```python
from build123d import *

# Parameters (mm, degrees)
SKETCH_1_R          = 32.5
SKETCH_1_R_2        = 13.625
SKETCH_1_R_3        = 2
SKETCH_1_R_4        = 1.65
SKETCH_1_R_5        = 1.4
EXTRUDE_1_DEPTH     = 4
SKETCH_2_R          = 1
CUT_EXTRUDE_1_DEPTH = 10


with BuildPart() as part:
    # 草图1 → 凸台-拉伸1 (new body)
    with BuildSketch(Plane.XY):
        with Locations((-0.261189045, 0.652972612)):
            Circle(SKETCH_1_R)
        with Locations((-0.261189045, 0.652972612)):
            Circle(SKETCH_1_R_2, mode=Mode.SUBTRACT)
        with Locations((-0.261189045, -27.347027388)):
            Circle(SKETCH_1_R_3, mode=Mode.SUBTRACT)
        with Locations((-26.890771501, -7.999503231)):
            Circle(SKETCH_1_R_3, mode=Mode.SUBTRACT)
        with Locations((-16.719176109, 23.305448454)):
            Circle(SKETCH_1_R_4, mode=Mode.SUBTRACT)
        with Locations((16.196798019, 23.305448454)):
            Circle(SKETCH_1_R_3, mode=Mode.SUBTRACT)
        with Locations((26.368393412, -7.999503231)):
            Circle(SKETCH_1_R_3, mode=Mode.SUBTRACT)
        with Locations((-12.016894091, -15.527367276)):
            Circle(SKETCH_1_R_5, mode=Mode.SUBTRACT)
        with Locations((-19.282319371, 6.833312499)):
            Circle(SKETCH_1_R_5, mode=Mode.SUBTRACT)
        with Locations((-0.261189045, 20.652972612)):
            Circle(SKETCH_1_R_5, mode=Mode.SUBTRACT)
        with Locations((18.759941281, 6.833312499)):
            Circle(SKETCH_1_R_5, mode=Mode.SUBTRACT)
        with Locations((11.494516001, -15.527367276)):
            Circle(SKETCH_1_R_5, mode=Mode.SUBTRACT)
    extrude(amount=EXTRUDE_1_DEPTH)

    # 草图2 → 切除-拉伸1 (cut)
    with BuildSketch(Plane.XY.offset(4)):
        with Locations((-13.870533326, 0)):
            Circle(SKETCH_2_R)
        with Locations((-32.761189045, 0.652972612)):
            Circle(SKETCH_2_R)
    extrude(amount=-CUT_EXTRUDE_1_DEPTH, mode=Mode.SUBTRACT)


solid = part.part
```
Can you work these out from the model? Positions are in its coordinate system, mm. A direction names the side the tool comes from. Coordinates: 2 decimals unless noted, no trailing zeros. Order: outer loops, then holes, each group sorted by start corner. A loop starts at its lowest first (then second) coordinate and runs counter-clockwise, first axis right, second up.
1. I need wall thicknesses on line 1 (Y direction, x = -0.5, z = 0.95); line 2 (X direction, y = -15, z = 3.65); line 3 (Y direction, x = -12, z = 2.6). Which ranges of each line are inside material? Lowest first, please.
2. Thinking about a two-plate mould opening in Y: for faces 3 (the face through (24.37, -7.91, 1.97)), 4 (the face through (-0.7, -13.3, 4)), 5 (the face through (-0.7, -29.3, 2)), which applies, +Y half, -Y half, draft (parallel to the pull), parting line (faces both ways), or undercut?
3. I'm going to push flat-ended pins straight in: pin 1 (1 mm diameter, centred on x = -10, z = 2, fed in from -Y); pin 2 (1 mm diameter, centred on y = 25.5, z = 1.5, fed in from +X); pin 3 (2 mm diameter, centred on x = -16.72, y = 23.31, fed in from +Z); pin 4 (1 mm diameter, centred on y = 23.5, z = 1.5, fed in from -X). Where does each tip first touch, or does it pass through?
4. If we section it at B-B (y = 3): Please give me the cut outline in (x, z).
5. If we section it at A-A (x = 16): Please give me the cut outline in (y, z).
6. If we section it at C-C (z = 0.7): Give the number of separate pieces and of enclosed holes in the cut face, then the cut area to 3 significant figures.
7. For faces 1 (the face through (-31.76, 0.63, 2.03)), 2 (the face through (-14.87, -0.03, 2.03)), which set-ups out of +Z, -Z, +X, -X, +Y, -Y let a thin tool reach every point of the face, with its end or its side?
8. If we section it at D-D (y = -9): Please give me the cut outline in (x, z), then the cut area to 3 significant figures.
Entries:
1. line 1: y = -31.85 to -29.33, -25.36 to -12.97, 14.28 to 19.27, 22.03 to 33.15
1. line 2: x = -28.74 to -13.31, -10.72 to 10.2, 12.79 to 28.22
1. line 3: y = -29.65 to -16.93, -14.13 to -6.26, 7.57 to 30.96
2. face 3: undercut
2. face 4: draft
2. face 5: undercut
3. pin 1: stops at y = -30.51
3. pin 2: stops at x = 21.27
3. pin 3: passes through
3. pin 4: stops at x = -23.86
4. outline: (-32.68, 0) - (-13.68, 0) - (-13.68, 4) - (-32.68, 4) - close; (13.16, 0) - (32.15, 0) - (32.15, 4) - (13.16, 4) - close
5. outline: (-27.49, 0) - (21.32, 0) - (21.32, 4) - (-27.49, 4) - close; (25.3, 0) - (28.79, 0) - (28.79, 4) - (25.3, 4) - close
6. separate pieces: 1
6. enclosed holes: 11
6. area: 2,640 mm2
7. face 1: +Z, -Z, -X
7. face 2: +Z, -Z
8. outline: (-31.29, 0) - (-28.62, 0) - (-28.62, 4) - (-31.29, 4) - close; (-25.16, 0) - (-9.88, 0) - (-9.88, 4) - (-25.16, 4) - close; (9.35, 0) - (24.64, 0) - (24.64, 4) - (9.35, 4) - close; (28.1, 0) - (30.77, 0) - (30.77, 4) - (28.1, 4) - close
8. area: 144 mm2
